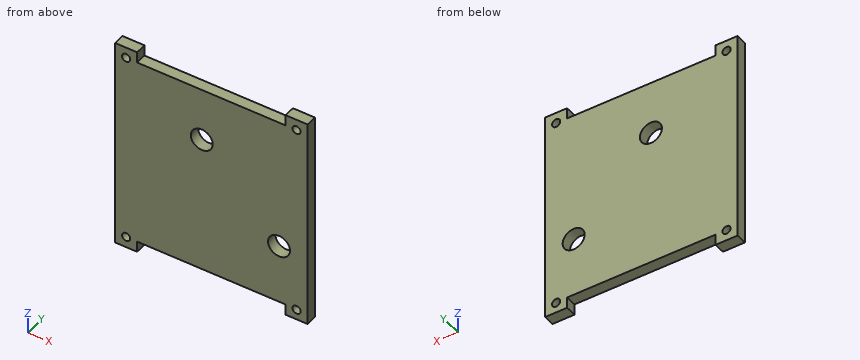
```python
from build123d import *

# Parameters (mm, degrees)
SKETCH1_R           = 0.75
BOSS_EXTRUDE1_DEPTH = 2
SKETCH2_R           = 2
CUT_EXTRUDE1_DEPTH  = 2


with BuildPart() as part:
    # Sketch1 → Boss-Extrude1 (new body)
    with BuildSketch(Plane(origin=(0, 4.390610578, 0), x_dir=(1, 0, 0), z_dir=(0, 1, 0))):
        Polygon((10.961043754, 31.726646364), (10.961043754, -7.273353636), (14.961043754, -7.273353636), (14.961043754, -5.273353636), (41.961043754, -5.273353636), (41.961043754, -7.273353636), (45.961043754, -7.273353636), (45.961043754, 31.726646364), (41.961043754, 31.726646364), (41.961043754, 29.726646364), (14.961043754, 29.726646364), (14.961043754, 31.726646364), align=None)
        with Locations(Location((12.961043754, -5.273353636, 0), (0, 0, 270))):
            Circle(SKETCH1_R, mode=Mode.SUBTRACT)
        with Locations(Location((43.961043754, -5.273353636, 0), (0, 0, 270))):
            Circle(SKETCH1_R, mode=Mode.SUBTRACT)
        with Locations(Location((43.961043754, 29.849185289, 0), (0, 0, 270))):
            Circle(SKETCH1_R, mode=Mode.SUBTRACT)
        with Locations(Location((12.961043754, 29.726646364, 0), (0, 0, 270))):
            Circle(SKETCH1_R, mode=Mode.SUBTRACT)
    extrude(amount=BOSS_EXTRUDE1_DEPTH)

    # Sketch2 → Cut-Extrude1 (cut)
    with BuildSketch(Plane(origin=(0, 6.390610578, 0), x_dir=(1, 0, 0), z_dir=(0, 1, 0))):
        with Locations(Location((26.718170314, 4.468036121, 0), (0, 0, 270))):
            Circle(SKETCH2_R)
        with Locations(Location((40.776506823, 18.857937171, 0), (0, 0, 270))):
            Circle(SKETCH2_R)
    extrude(amount=-CUT_EXTRUDE1_DEPTH, mode=Mode.SUBTRACT)


solid = part.part
```
CAD build for the part. Positions are in the model's coordinates, mm. Round coordinates to 2 decimals unless told otherwise and drop trailing zeros. Order: outer loops, then holes, each group sorted by start corner. A loop starts at its lowest first (then second) coordinate and runs counter-clockwise, first axis right, second up.
Q1. Slice it at A-A (y = 5.5). Write the cut outline in (x, z).
Q2. Wall check: L1, parallel to Z at x = 13, y = 6.25; L2, parallel to X at y = 5.5, z = -19; L3, parallel to Z at x = 31.5, y = 4.9. Give the ranges that are in metal, low to high.
Q3. Slice it at B-B (x = 41.5). Write the cut outline in (y, z).
Q4. Drop a flat-ended pin along its axis: pin 1 (1 mm diameter, centred on x = 23, y = 6, fed in from +Z). Give the stop position or say it passes through.
Q5. Slice it at C-C (x = 17.5). Write the cut outline in (y, z), and give its area (3 significant figures).
Results below:
1. outline: (10.96, -31.73) - (14.96, -31.73) - (14.96, -29.73) - (41.96, -29.73) - (41.96, -31.73) - (45.96, -31.73) - (45.96, 7.27) - (41.96, 7.27) - (41.96, 5.27) - (14.96, 5.27) - (14.96, 7.27) - (10.96, 7.27) - close; hole circle Ø1.5 at (12.96, -29.73); hole circle Ø1.5 at (12.96, 5.27); hole circle Ø4 at (26.72, -4.47); hole circle Ø4 at (40.78, -18.86); hole circle Ø1.5 at (43.96, -29.85); hole circle Ø1.5 at (43.96, 5.27)
2. L1: z = -31.73 to -30.48, -28.98 to 4.52, 6.02 to 7.27
2. L2: x = 10.96 to 38.78, 42.77 to 45.96
2. L3: z = -29.73 to 5.27
3. outline: (4.39, -29.73) - (6.39, -29.73) - (6.39, -20.72) - (4.39, -20.72) - close; (4.39, -16.99) - (6.39, -16.99) - (6.39, 5.27) - (4.39, 5.27) - close
4. pin 1: stops at z = 5.27
5. outline: (4.39, -29.73) - (6.39, -29.73) - (6.39, 5.27) - (4.39, 5.27) - close
5. area: 70.0 mm2
